Source: three-view drawing plus pictorial views. Frame: mm from the lowest corner of the part. A direction names the side the tool comes from. Give positions to 0.01 mm unless a question says otherwise; leave off trailing zeros. Order: outer loops, then holes, each group sorted by start corner. A loop starts at its lowest first (then second) coordinate and runs counter-clockwise, first axis right, second up. Notation, with made-up numbers: (-30.75, 87.5) - (6.25, 87.5) arc R12 ccw to (6.25, 106.5) - close; hole circle Ø1 at (73.5, 10.5). An arc over 180 degrees is marked (long way). Answer in a Markdown table with one row per item. Add a question column.
1. Section query D-D on y = 2.5. Return loops of the section in (x, z).
2. Section query A-A on z = 10.5. Return loops of the section in (x, y) (1 decimal), and give its area (3 significant figures).
3. Mould query, pull axis X, two halves, no side actions, for the marked faces 1, 2, 3 and 4. Classes: released by +X, released by -X, zero draft, split by the parting line, or undercut.
4. Contact query for flat-ended pins moving along their axis: pin 1 (0.9 mm diameter, centred on x = 12.5, y = 2, fed in from -Z); pin 2 (4 mm diameter, centred on x = 1.5, y = 10.5, fed in from +Z); pin 3 (4.5 mm diameter, centred on x = 9, y = 17, fed in from +Z) (1 decimal); pin 4 (4 mm diameter, centred on x = 7.5, z = 23, fed in from -Y). Output: stop coordinate, or through.
5. Section query B-B on z = 19. Return loops of the section in (x, y), and give its area (3 significant figures).
6. Section query C-C on x = 14. Count the separate pieces of the cut face and the enclosed holes in it, and give its area (3 significant figures).
7. Ray query, line 1 (Z direction, x = 12.35, y = 14); line 2 (X direction, y = 17, z = 25); line 3 (Y direction, x = 2.9, z = 29.5). Return the intervals inside material, ascending. Write a range as [from, to].
8. Access query for the marked faces 5, 6 and 7. Directions: +Z, -Z, +X, -X, +Y, -Y. A direction counts if a zero-diameter tool reaches every point of the face in a straight line with its end or side. Return the directions, or none.
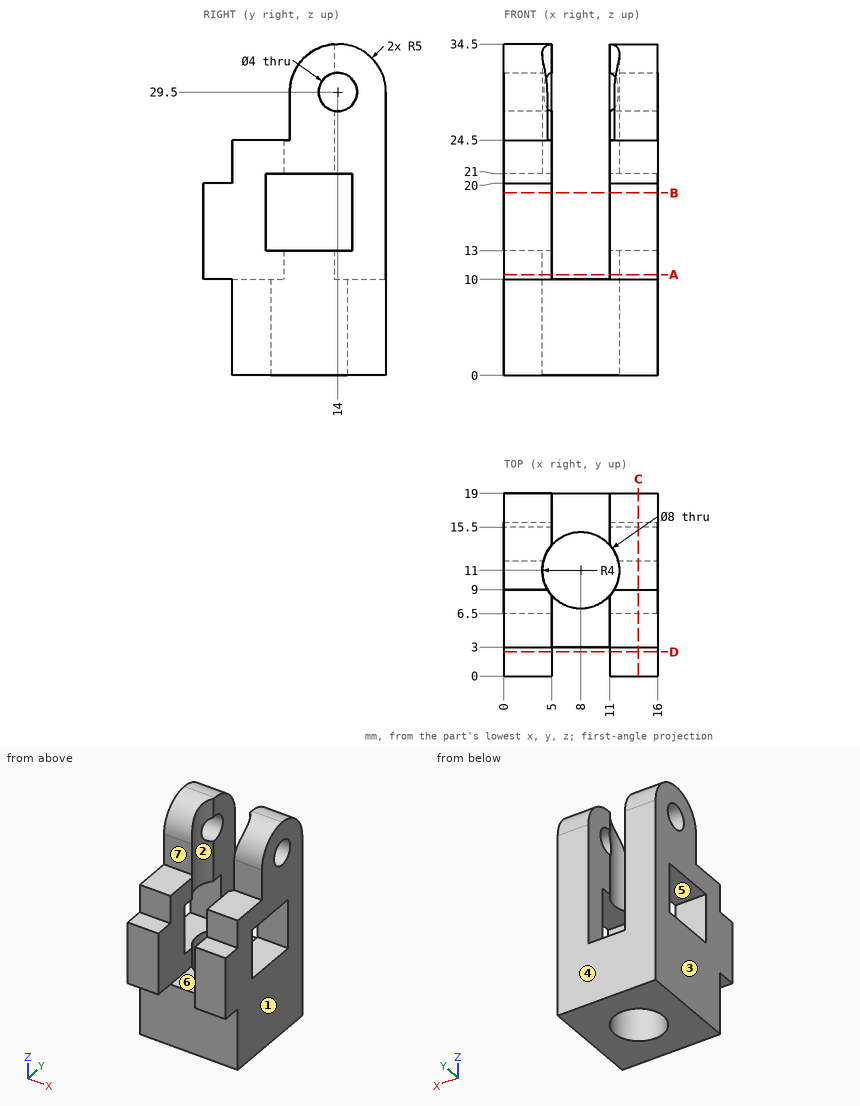
Answer:
| question | item | result |
|---|---|---|
| 1 | outline | (0, 10) - (5, 10) - (5, 20) - (0, 20) - close; (11, 10) - (16, 10) - (16, 20) - (11, 20) - close |
| 2 | outline | (0, 0) - (5, 0) - (5, 8.4) arc R4 cw to (5, 13.6) - (5, 19) - (0, 19) - close; (11, 0) - (16, 0) - (16, 19) - (11, 19) - (11, 13.6) arc R4 cw to (11, 8.4) - close |
| 2 | area | 183 mm² |
| 3 | face 1 | released by +X |
| 3 | face 2 | undercut |
| 3 | face 3 | released by -X |
| 3 | face 4 | zero draft |
| 4 | pin 1 | stops at z = 10 |
| 4 | pin 2 | stops at z = 34.27 |
| 4 | pin 3 | stops at z = 34.1 |
| 4 | pin 4 | passes through |
| 5 | outline | (0, 0) - (5, 0) - (5, 6.5) - (0, 6.5) - close; (0, 15.5) - (5, 15.5) - (5, 19) - (0, 19) - close; (11, 0) - (16, 0) - (16, 6.5) - (11, 6.5) - close; (11, 15.5) - (16, 15.5) - (16, 19) - (11, 19) - close |
| 5 | area | 100 mm² |
| 6 | separate pieces | 1 |
| 6 | enclosed holes | 2 |
| 6 | area | 427 mm² |
| 7 | line 1 | z = [0, 13], [21, 27.5], [31.5, 34.5] |
| 7 | line 2 | x = [0, 5], [11, 16] |
| 7 | line 3 | y = [9, 12], [16, 19] |
| 8 | face 5 | +X, -X |
| 8 | face 6 | +Z, +Y, -Y |
| 8 | face 7 | +Z, +X, -X, -Y |
